Input: part model. Units: mm. Frame: model coordinates. Face numbers are marked on the shaded views. A direction names the side the tool comes from. Give positions to 0.01 mm unless a question says otherwise; leave off trailing zeros. Loops run counter-clockwise (first coordinate to the right, second up) from the corner with the lowest first, then second, coordinate; pieces in that order, holes last. Notation, with made-up numbers: (-18, 37.25) - (8, 37.25) arc R19 cw to (8, 59.25) - close; hole circle Ø2 at (72.5, 67). An arc over 180 degrees is marked (long way). Answer as a JSON object with one key per item and string values.
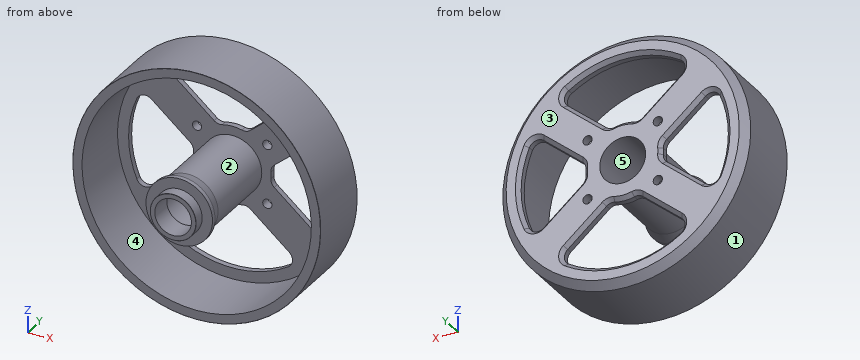
from build123d import *

# Parameters (mm, degrees)
HOLE_WIZARD_M3_1_D  = 2.5
CUT_EXTRUDE_1_DEPTH = 10
CHAMFER_1_SIZE      = 2
FILLET_1_R          = 2.5
CHAMFER_2_SIZE      = 1
CHAMFER_3_SIZE      = 0.05
CHAMFER_4_SIZE      = 0.05


with BuildPart() as part:
    # 草图6 → 旋转1 (revolve)
    with BuildSketch(Plane.XY, mode=Mode.PRIVATE) as revolve_1_sk:
        Polygon((33.5, 0), (33.5, 19.8), (6.2, 19.8), (6.2, -5.621788423), (4.95, -5.621788423), (4.95, -11.5), (6.2, -11.5), (6.2, -8.5), (9, -8.5), (9, -7.3), (8, -4), (8, 17.3), (31, 17.3), (31, 0), align=None)
    revolve(revolve_1_sk.sketch.rotate(Axis((0, 0, 0), (0, 1, 0)), 90), axis=Axis((0, 0, 0), (0, 1, 0)))

    # M3 螺纹孔1 (through all)
    with Locations(Plane(origin=(0, 19.8, 0), x_dir=(1, 0, 0), z_dir=(0, 1, 0))):
        with Locations((9.5, -8), (-9.5, -8), (-9.5, 8), (9.5, 8)):
            Hole(HOLE_WIZARD_M3_1_D / 2)

    # 草图11 → 切除-拉伸1 (cut)
    with BuildSketch(Plane(origin=(0, 19.8, 0), x_dir=(1, 0, 0), z_dir=(0, 1, 0))):
        with BuildLine():
            Line((17.852590074, 21.570466561), (3.841817237, 9.771921015))
            ThreePointArc((3.841817237, 9.771921015), (0, 10.5), (-3.841817237, 9.771921015))
            Line((-3.841817237, 9.771921015), (-17.852590074, 21.570466561))
            ThreePointArc((-17.852590074, 21.570466561), (0, 28), (17.852590074, 21.570466561))
        make_face()
        with BuildLine():
            Line((24.293947531, -13.92135458), (10.283174695, -2.122809033))
            ThreePointArc((10.283174695, -2.122809033), (10.5, 0), (10.283174695, 2.122809033))
            Line((10.283174695, 2.122809033), (24.293947531, 13.92135458))
            ThreePointArc((24.293947531, 13.92135458), (28, 0), (24.293947531, -13.92135458))
        make_face()
        with BuildLine():
            Line((17.852590074, -21.570466561), (3.841817237, -9.771921015))
            ThreePointArc((3.841817237, -9.771921015), (0, -10.5), (-3.841817237, -9.771921015))
            Line((-3.841817237, -9.771921015), (-17.852590074, -21.570466561))
            ThreePointArc((-17.852590074, -21.570466561), (0, -28), (17.852590074, -21.570466561))
        make_face()
        with BuildLine():
            Line((-10.283174695, 2.122809033), (-24.293947531, 13.92135458))
            ThreePointArc((-24.293947531, 13.92135458), (-28, 0), (-24.293947531, -13.92135458))
            Line((-24.293947531, -13.92135458), (-10.283174695, -2.122809033))
            ThreePointArc((-10.283174695, -2.122809033), (-10.5, 0), (-10.283174695, 2.122809033))
        make_face()
    extrude(amount=-CUT_EXTRUDE_1_DEPTH, mode=Mode.SUBTRACT)

    # 倒角1
    chamfer_1_edges = [part.edges().sort_by_distance(p)[0] for p in [
        (0, 19.8, 33.5),
    ]]
    chamfer(chamfer_1_edges, length=CHAMFER_1_SIZE)

    # 圆角1
    fillet_1_edges = [part.edges().sort_by_distance(p)[0] for p in [
        (17.852590074, 18.55, 21.570466561),
        (-17.852590074, 18.55, 21.570466561),
        (-3.841817237, 18.55, 9.771921015),
        (3.841817237, 18.55, 9.771921015),
        (24.293947531, 18.55, -13.92135458),
        (24.293947531, 18.55, 13.92135458),
        (10.283174695, 18.55, 2.122809033),
        (10.283174695, 18.55, -2.122809033),
        (-24.293947531, 18.55, 13.92135458),
        (-24.293947531, 18.55, -13.92135458),
        (-10.283174695, 18.55, -2.122809033),
        (-10.283174695, 18.55, 2.122809033),
        (-17.852590074, 18.55, -21.570466561),
        (17.852590074, 18.55, -21.570466561),
        (3.841817237, 18.55, -9.771921015),
        (-3.841817237, 18.55, -9.771921015),
    ]]
    fillet(fillet_1_edges, radius=FILLET_1_R)

    # 倒角2
    chamfer_2_edges = [part.edges().sort_by_distance(p)[0] for p in [
        (0, 19.8, 28),
        (-10.161632191, 19.8, 15.093870449),
        (0, 19.8, 10.5),
        (10.161632191, 19.8, 15.093870449),
        (28, 19.8, 0),
        (16.602989649, 19.8, 7.444758468),
        (10.5, 19.8, 0),
        (16.602989649, 19.8, -7.444758468),
        (0, 19.8, -28),
        (10.161632191, 19.8, -15.093870449),
        (-10.161632191, 19.8, -15.093870449),
        (0, 19.8, -10.5),
        (-16.602989649, 19.8, 7.444758468),
        (-28, 19.8, 0),
        (-10.5, 19.8, 0),
        (-16.602989649, 19.8, -7.444758468),
        (-16.306405676, 19.8, 21.595078628),
        (-3.841486524, 19.8, 10.13784984),
        (3.841486524, 19.8, 10.13784984),
        (16.306405676, 19.8, 21.595078628),
        (24.055073585, 19.8, 12.393535487),
        (10.643709543, 19.8, 2.060210005),
        (10.643709543, 19.8, -2.060210005),
        (24.055073585, 19.8, -12.393535487),
        (16.306405676, 19.8, -21.595078628),
        (-16.306405676, 19.8, -21.595078628),
        (-3.841486524, 19.8, -10.13784984),
        (3.841486524, 19.8, -10.13784984),
        (-24.055073585, 19.8, 12.393535487),
        (-10.643709543, 19.8, 2.060210005),
        (-10.643709543, 19.8, -2.060210005),
        (-24.055073585, 19.8, -12.393535487),
    ]]
    chamfer(chamfer_2_edges, length=CHAMFER_2_SIZE)

    # 倒角3
    chamfer_3_edges = [part.edges().sort_by_distance(p)[0] for p in [
        (0, 0, 33.5),
    ]]
    chamfer(chamfer_3_edges, length=CHAMFER_3_SIZE)

    # 倒角4
    chamfer_4_edges = [part.edges().sort_by_distance(p)[0] for p in [
        (0, -11.5, 6.2),
    ]]
    chamfer(chamfer_4_edges, length=CHAMFER_4_SIZE)


solid = part.part
Item 1: Access query for the marked faces 4 and 5. Directions: +Z, -Z, +X, -X, +Y, -Y. A direction counts if a zero-diameter tool reaches every point of the face in a straight line with its end or side. Return the directions, or none.
Geometry check:
{"face 4": "-Y", "face 5": "+Y"}
Item 2: Contact query for flat-ended pins moving along their axis: P1, Ø3, axis at x = 9.5, y = 14, coming from the +Z side; P2, Ø7.5, axis at x = 0, z = 0, coming from the -Y side; P3, Ø3, axis at x = 9.5, z = 8, coming from the -Y side; P4, Ø12, axis at y = 16, z = 8, coming from the -X side. Output: stop coordinate, or through.
Geometry check:
{"P1": "stops at z = 32.53", "P2": "passes through", "P3": "stops at y = 17.3", "P4": "stops at x = -33.44"}
Item 3: Mould query, pull axis X, two halves, no side actions, for the marked faces 1, 2 and 3. Classes: released by +X, released by -X, zero draft, split by the parting line, or undercut.
Geometry check:
{"face 1": "split by the parting line", "face 2": "undercut", "face 3": "zero draft"}
Item 4: Material intervals for line 1 (X direction, y = 7, z = 0); line 2 (X direction, y = 19, z = -8); line 3 (Z direction, x = 9.5, y = 19.15), sorted ascending. Write a range as [from, to].
Geometry check:
{"line 1": "x = [-33.5, -31], [-8, -6.2], [6.2, 8], [31, 33.5]", "line 2": "x = [-31.29, -27.04], [-16.95, -10.75], [-8.25, 8.25], [10.75, 16.95], [27.04, 31.29]", "line 3": "z = [-30.71, -26.71], [-14.08, -9.25], [-6.75, 6.75], [9.25, 14.08], [26.71, 30.71]"}
Item 5: Cut plane A-A (y = 4.5). Return loops of the section in (x, z), then the cut area to 3 significant figures.
Geometry check:
{"outline": "circle Ø67 at (0, 0); circle Ø16 at (0, 0); hole circle Ø62 at (0, 0); hole circle Ø12.4 at (0, 0)", "area": "587 mm2"}
